Input: part model. Units: mm. Frame: model coordinates. Coordinates: 2 decimals unless noted, no trailing zeros. Write each loop counter-clockwise with the first axis right and the second up, starting at its lowest first coordinate (ties: lowest second). Pieces come first, ordered by that corner, then holes. Notation, with made-up numbers: (12, 84.25) - (37, 84.25) arc R27 ccw to (37, 122.25) - close; hole circle Ø4 at (-23.5, 22.5). An arc over 180 degrees is marked (long way). Use a Markdown table: item, result. Add a question column.
Q1. Section query A-A (x = 22). Return the cut outline in (y, z).
Q2. Material intervals for probe 1 along X at (y, z) = (1.5, -2.2); probe 2 along Z at (x, y) = (36, 2.5); probe 3 along X at (y, z) = (2.25, -1.35), sorted ascending. Write a range as from..to.
Q3. Pin query (flat end, axial travel): P1, Ø2, axis at x = -12, z = -1, coming from the -Y side. Return the tip coordinate at first contact, or that it passes through.
from build123d import *

# Parameters (mm, degrees)
CHAMFER1_SIZE           = 0.5
SKETCH2_W               = 2
SKETCH2_H               = 6
CUT_EXTRUDE1_DEPTH      = 40.3098
CUT_EXTRUDE1_DEPTH_BACK = 18.9666


with BuildPart() as part:
    # Sketch1 → Revolve1 (revolve)
    with BuildSketch(Plane.XY):
        Polygon((-17.9666, 0), (39.3098, 0), (39.3098, 3), (37.3098, 3), (36.5732, 3), (17.7732, 3), (17.7732, 2.5), (17.0366, 2.5), (17.0366, 3), (0.7366, 3), (0.7366, 2.5), (0, 2.5), (0, 3), (-15.23, 3), (-15.23, 2.5), (-15.9666, 2.5), (-15.9666, 3), (-17.9666, 3), align=None)
    revolve(axis=Axis((-17.9666, 0, 0), (-1, 0, 0)))

    # Chamfer1
    chamfer1_edges = [part.edges().sort_by_distance(p)[0] for p in [
        (39.3098, -3, 0),
        (-17.9666, -3, 0),
    ]]
    chamfer(chamfer1_edges, length=CHAMFER1_SIZE)

    # Sketch2 → Cut-Extrude1 (cut, two sides)
    with BuildSketch(Plane(origin=(0, 0, 0), x_dir=(0, 0, -1), z_dir=(1, 0, 0))) as cut_extrude1_sk:
        with Locations((-3.5, 0)):
            Rectangle(SKETCH2_W, SKETCH2_H)
    extrude(amount=CUT_EXTRUDE1_DEPTH, mode=Mode.SUBTRACT)
    extrude(cut_extrude1_sk.sketch, amount=-CUT_EXTRUDE1_DEPTH_BACK, mode=Mode.SUBTRACT)


solid = part.part
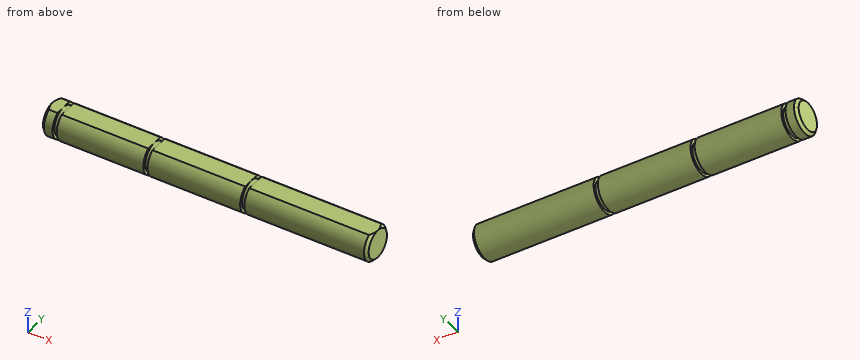
Values follow:
| question | item | result |
|---|---|---|
| 1 | outline | (-1.66, 2.5) arc R3 ccw (long way) to (1.66, 2.5) - close |
| 2 | probe 1 | -17.8..-15.97, -15.23..0, 0.74..17.04, 17.77..39.15 |
| 2 | probe 2 | -1.66..1.66 |
| 2 | probe 3 | -17.84..-15.97, -15.23..0, 0.74..17.04, 17.77..39.19 |
| 3 | P1 | y = -3 |
